Check sheet for the modelled part. Datum: model origin and axes. Units: mm. Face numbers are marked on the shaded views. Round coordinates to 2 decimals unless told otherwise and drop trailing zeros. Loops run counter-clockwise (first coordinate to the right, second up) from the corner with the lowest first, then second, coordinate; pieces in that order, holes last. Notation, with made-up numbers: M -16.5,45 L 2.5,45 A29 cw 2.5,76 Z; hole C -30.75,-36.75 d6. An arc over 180 degrees is marked long. One line per question, with ' | ' between items. Start each with the question number.
(1) Section check C-C (z = 120.02). Record the boundary of the cut face in (x, y).
(2) Section check B-B (x = -8.5). Record the boundary of the cut face in (y, z), and give its area (3 significant figures).
(3) Go/stop test with flat-tipped pins: P1, Ø9.5, axis at x = -61.15, z = 17.55, coming from the -Y side; P2, Ø3.5, axis at x = -8.5, z = 120.02, coming from the +Y side; P3, Ø1.9, axis at x = -8.5, z = 120.02, coming from the -Y side; P4, Ø5, axis at x = 12.87, z = 15.05, coming from the +Y side. Record where each tip stops, or that it passes through.
(4) Section check D-D (x = -61.15). Record the boundary of the cut face in (y, z), and give its area (3 significant figures).
(5) Section check A-A (y = -1.5). Record the boundary of the cut face in (x, z).
(6) Thickness scan on probe 1 along Z at (x, y) = (8.5, -1.85); probe 2 along Z at (x, y) = (12.87, 3.95); probe 3 along X at (y, z) = (0.15, 11.09). Record the ranges inside material, lowest first. Write a range as [from, to].
(7) Draft check along X on the marked faces 1 and 2. Enter one of: +X half, -X half, draft (parallel to the pull), parting line (faces both ways), or undercut.
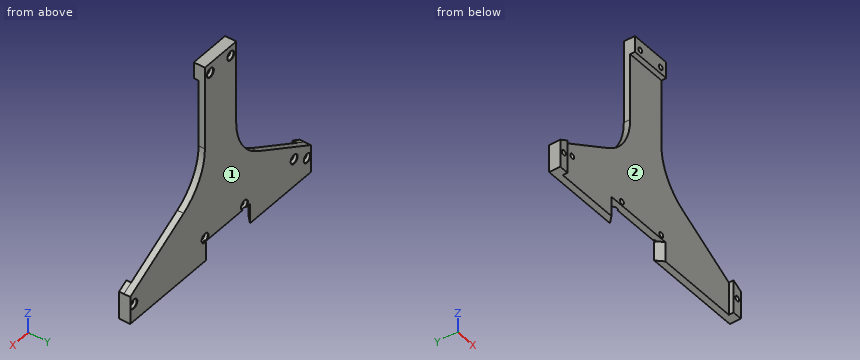
```python
from build123d import *

# Parameters (mm, degrees)
BOSS_EXTRU_1_DEPTH       = 4
BOSS_EXTRU_6_DEPTH       = 3
ESQUISSE22_W             = 26
ESQUISSE22_H             = 11.3
BOSS_EXTRU_7_DEPTH       = 3
ENL_V_MAT_EXTRU_9_DEPTH  = 12.6
ENL_V_MAT_EXTRU_10_REACH = 149.934
ESQUISSE23_W             = 26
ESQUISSE23_H             = 1


# Read off the part's stored shape, not the designer's step: Fraisage pour vis à tête fraisée à 6 pans creux M31
with BuildPart() as part:
    # Esquisse1 → Boss.-Extru.1 (new body)
    with BuildSketch(Plane(origin=(0, 0, 0), x_dir=(1, 0, 0), z_dir=(0, 1, 0))):
        with BuildLine():
            Line((-13, -127.32), (-13, -73.32))
            ThreePointArc((-13, -73.32), (-17.738590223, -55.734577677), (-30.671261616, -42.910875941))
            Line((-30.671261616, -42.910875941), (-75, -17.65))
            Line((-75, -17.65), (-75, 0))
            Line((-75, 0), (75, 0))
            Line((75, 0), (75, -17.65))
            Line((75, -17.65), (30.671261616, -42.910875941))
            ThreePointArc((30.671261616, -42.910875941), (17.738590223, -55.734577677), (13, -73.32))
            Line((13, -73.32), (13, -127.32))
            Line((13, -127.32), (-13, -127.32))
        make_face()
    extrude(amount=BOSS_EXTRU_1_DEPTH)

    # Esquisse21 → Boss.-Extru.6 (add)
    with BuildSketch(Plane(origin=(0, 0, 0), x_dir=(-1, 0, 0), z_dir=(0, -1, 0))):
        Polygon((75, 0), (69, 0), (69, -21.069119541), (75, -17.65), align=None)
        Polygon((-75, 0), (-69, 0), (-69, -21.069119541), (-75, -17.65), align=None)
    extrude(amount=BOSS_EXTRU_6_DEPTH)

    # Esquisse22 → Boss.-Extru.7 (add)
    with BuildSketch(Plane.XZ):
        with Locations((0, 121.67)):
            Rectangle(ESQUISSE22_W, ESQUISSE22_H)
    extrude(amount=BOSS_EXTRU_7_DEPTH)

    # Fraisage pour vis _ t_te frais_e _ 6 2 → Fraisage pour vis à tête fraisée à 6 pans creux M31 (revolve, cut)
    with BuildSketch(Plane(origin=(8.5, 0, 120.02), x_dir=(1, 0, 0), z_dir=(0, 0, 1))):
        Polygon((0, -3), (1.6, -3), (1.6, 2.3), (2.9, 3.6), (2.9, 4), (0, 4), align=None)
    revolve(axis=Axis((8.5, 0, 120.02), (0, 1, 0)), mode=Mode.SUBTRACT)

    # Fraisage pour vis _ t_te frais_e _ 6 3 o → Fraisage pour vis _ t_te frais_e _ 6 3 (revolve, cut)
    with BuildSketch(Plane(origin=(-8.5, 0, 120.02), x_dir=(1, 0, 0), z_dir=(0, 0, 1))):
        Polygon((0, -3), (1.6, -3), (1.6, 2.3), (2.9, 3.6), (2.9, 4), (0, 4), align=None)
    revolve(axis=Axis((-8.5, 0, 120.02), (0, 1, 0)), mode=Mode.SUBTRACT)

    # Fraisage pour vis _ t_te frais_e _ 6 4 o → Fraisage pour vis _ t_te frais_e _ 6 4 (revolve, cut)
    with BuildSketch(Plane(origin=(-61.15, 0, 17.55), x_dir=(1, 0, 0), z_dir=(0, 0, 1))):
        Polygon((0, 0), (1.6, 0), (1.6, 2.3), (2.9, 3.6), (2.9, 4), (0, 4), align=None)
    revolve(axis=Axis((-61.15, 0, 17.55), (0, 1, 0)), mode=Mode.SUBTRACT)

    # Fraisage pour vis _ t_te frais_e _ 6 5 o → Fraisage pour vis _ t_te frais_e _ 6 5 (revolve, cut)
    with BuildSketch(Plane(origin=(-72, 0, 11.09), x_dir=(1, 0, 0), z_dir=(0, 0, 1))):
        Polygon((0, -3), (1.6, -3), (1.6, 2.3), (2.9, 3.6), (2.9, 4), (0, 4), align=None)
    revolve(axis=Axis((-72, 0, 11.09), (0, 1, 0)), mode=Mode.SUBTRACT)

    # Fraisage pour vis _ t_te frais_e _ 6 6 o → Fraisage pour vis _ t_te frais_e _ 6 6 (revolve, cut)
    with BuildSketch(Plane(origin=(72, 0, 11.09), x_dir=(1, 0, 0), z_dir=(0, 0, 1))):
        Polygon((0, -3), (1.6, -3), (1.6, 2.3), (2.9, 3.6), (2.9, 4), (0, 4), align=None)
    revolve(axis=Axis((72, 0, 11.09), (0, 1, 0)), mode=Mode.SUBTRACT)

    # Fraisage pour vis _ t_te frais_e _ 6 7 o → Fraisage pour vis _ t_te frais_e _ 6 7 (revolve, cut)
    with BuildSketch(Plane(origin=(12.87, 0, 15.05), x_dir=(1, 0, 0), z_dir=(0, 0, 1))):
        Polygon((0, 0), (1.6, 0), (1.6, 2.3), (2.9, 3.6), (2.9, 4), (0, 4), align=None)
    revolve(axis=Axis((12.87, 0, 15.05), (0, 1, 0)), mode=Mode.SUBTRACT)

    # Fraisage pour vis _ t_te frais_e _ 6 8 o → Fraisage pour vis _ t_te frais_e _ 6 8 (revolve, cut)
    with BuildSketch(Plane(origin=(-19.84, 0, 15.05), x_dir=(1, 0, 0), z_dir=(0, 0, 1))):
        Polygon((0, 0), (1.6, 0), (1.6, 2.3), (2.9, 3.6), (2.9, 4), (0, 4), align=None)
    revolve(axis=Axis((-19.84, 0, 15.05), (0, 1, 0)), mode=Mode.SUBTRACT)

    # Esquisse16 → Enlèv. mat.-Extru.9 (cut)
    with BuildSketch(Plane(origin=(0, 0, 0), x_dir=(-1, 0, 0), z_dir=(0, 0, -1))):
        Polygon((28.5, 0), (24.5, 4), (-12.25, 4), (-16.25, 0), align=None)
    extrude(amount=-ENL_V_MAT_EXTRU_9_DEPTH, mode=Mode.SUBTRACT)

    # Esquisse23 → Enlèv. mat.-Extru.10 (cut, up to next)
    with BuildSketch(Plane(origin=(0, 4, 0), x_dir=(1, 0, 0), z_dir=(0, 1, 0)), mode=Mode.PRIVATE) as enl_v_mat_extru_10_sk1:
        with Locations((0, -126.82)):
            Rectangle(ESQUISSE23_W, ESQUISSE23_H)
    enl_v_mat_extru_10_tool1 = extrude(enl_v_mat_extru_10_sk1.sketch, amount=-ENL_V_MAT_EXTRU_10_REACH, mode=Mode.PRIVATE) & part.part
    add(enl_v_mat_extru_10_tool1.solids().sort_by_distance((0, 4, 126.82))[0], mode=Mode.SUBTRACT)


solid = part.part
```
The answers:
1) outline: M -13,-3 L -10.1,-3 L -10.1,2.3 L -11.4,3.6 L -11.4,4 L -13,4 Z; M -6.9,-3 L 6.9,-3 L 6.9,2.3 L 5.6,3.6 L 5.6,4 L -5.6,4 L -5.6,3.6 L -6.9,2.3 Z; M 10.1,-3 L 13,-3 L 13,4 L 11.4,4 L 11.4,3.6 L 10.1,2.3 Z
2) outline: M -3,116.02 L 0,116.02 L 0,12.6 L 4,12.6 L 4,117.12 L 3.6,117.12 L 2.3,118.42 L -3,118.42 Z; M -3,121.62 L 2.3,121.62 L 3.6,122.92 L 4,122.92 L 4,126.32 L -3,126.32 Z | area: 461 mm²
3) P1: y = 0 | P2: y = 2.45 | P3: through | P4: y = 3.2
4) outline: M 0,0 L 4,0 L 4,14.65 L 3.6,14.65 L 2.3,15.95 L 0,15.95 Z; M 0,19.15 L 2.3,19.15 L 3.6,20.45 L 4,20.45 L 4,25.54 L 0,25.54 Z | area: 86.6 mm²
5) outline: M -75,0 L -69,0 L -69,21.07 L -75,17.65 Z; M -13,116.02 L 13,116.02 L 13,126.32 L -13,126.32 Z; M 69,0 L 75,0 L 75,17.65 L 69,21.07 Z; hole C -72,11.09 d3.2; hole C -8.5,120.02 d3.2; hole C 8.5,120.02 d3.2; hole C 72,11.09 d3.2
6) probe 1: [116.02, 118.42], [121.62, 126.32] | probe 2: [0, 12.15], [17.95, 126.32] | probe 3: [-75, -73.6], [-70.4, -28.35], [16.1, 70.4], [73.6, 75]
7) face 1: draft | face 2: undercut
